Autodesk Inventor part; units mm, degrees
ref_plane "YZ Plane" through (0, 0, 0) normal (1, 0, 0) x (0, 1, 0)
ref_plane "XZ Plane" through (0, 0, 0) normal (0, 1, 0) x (-1, 0, 0)
ref_plane "XY Plane" through (0, 0, 0) normal (0, 0, 1) x (1, 0, 0)
sketch "Skizze1" plane through (0, 0, 0) normal (0, 1, 0) x (-1, 0, 0)
  line L0 (0, 0) -> (15, 0)
  line L1 (15, 0) -> (15, -17.5)
  line L2 (15, -17.5) -> (40, -17.5)
  line L3 (40, -17.5) -> (40, -47.5)
  line L4 (40, -47.5) -> (15, -47.5)
  line L5 (15, -47.5) -> (15, -65)
  line L6 (15, -65) -> (0, -65)
  line L7 (0, -65) -> (0, 0)
  dimension "d0" = 65
  dimension "d1" = 30
  dimension "d2" = 15
  dimension "d3" = 40
  dimension "d6" = 25
extrude "Extrusion3" add sketch "Skizze1" along normal blind 12
sketch "Skizze5" plane through (0, 0, 0) normal (0, -1, 0) x (1, 0, 0)
  line L0 (-7.5, -58) -> (-7.5, -43) construction
  line L1 (-4.95, -58) -> (-4.95, -43)
  line L2 (-10.05, -43) -> (-10.05, -58)
  arc A0 (-10.05, -58) -> (-4.95, -58) centre (-7.5, -58) ccw
  arc A1 (-4.95, -43) -> (-10.05, -43) centre (-7.5, -43) ccw
  line L3 (-7.5, -22) -> (-7.5, -7) construction
  line L4 (-4.95, -22) -> (-4.95, -7)
  line L5 (-10.05, -7) -> (-10.05, -22)
  arc A2 (-10.05, -22) -> (-4.95, -22) centre (-7.5, -22) ccw
  arc A3 (-4.95, -7) -> (-10.05, -7) centre (-7.5, -7) ccw
  line L6 (0, -65) -> (-15, -65)
  line L7 (-15, 0) -> (0, 0)
  line L8 (-15, -65) -> (-15, -47.5)
  line L9 (0, 0) -> (0, -65)
  point P0 (-7.5, -50.5)
  point P1 (-7.5, -14.5)
  dimension "d52" = 5.1
  dimension "d53" = 5.1
  dimension "d54" = 15
  dimension "d55" = 15
  dimension "d56" = 7
  dimension "d58" = 7
  dimension "d59" = 15
  dimension "d60" = 7.5
  dimension "d76" = 36
extrude "Extrusion5" cut sketch "Skizze5" against normal through all
sketch "Skizze6" plane through (0, 0, 0) normal (0, -1, 0) x (1, 0, 0)
  line L0 (-7.5, -58) -> (-7.5, -43) construction
  line L1 (-2.5, -58) -> (-2.5, -43)
  line L2 (-12.5, -43) -> (-12.5, -58)
  arc A0 (-12.5, -58) -> (-2.5, -58) centre (-7.5, -58) ccw
  arc A1 (-2.5, -43) -> (-12.5, -43) centre (-7.5, -43) ccw
  line L3 (-7.5, -22) -> (-7.5, -7) construction
  line L4 (-2.5, -22) -> (-2.5, -7)
  line L5 (-12.5, -7) -> (-12.5, -22)
  arc A2 (-12.5, -22) -> (-2.5, -22) centre (-7.5, -22) ccw
  arc A3 (-2.5, -7) -> (-12.5, -7) centre (-7.5, -7) ccw
  line L6 (-15, 0) -> (0, 0)
  line L7 (0, 0) -> (0, -65)
  point P0 (-7.5, -50.5)
  point P1 (-7.5, -14.5)
  dimension "d63" = 10
  dimension "d64" = 10
  dimension "d65" = 15
  dimension "d66" = 15
  dimension "d67" = 7
  dimension "d68" = 7.5
  dimension "d69" = 7.5
  dimension "d70" = 7
extrude "Extrusion6" cut sketch "Skizze6" against normal blind 5
fillet "Rundung4" radius 7.5 6 edges at (-15, 6, -65) (0, 6, -65) (0, 6, 0) (-15, 6, 0) (-15, 6, -17.5) (-15, 6, -47.5)
fillet "Rundung5" radius 15 2 edges at (-40, 6, -47.5) (-40, 6, -17.5)
sketch "Skizze7" plane through (0, 0, 0) normal (0, -1, 0) x (1, 0, 0)
  circle A0 centre (-30.5, -32.5) radius 3.7991
  point P0 (0, 0)
  dimension "d77" = 32.5
  dimension "d78" = 30.5
hole "Bohrung1" at (-30.5, 0, -32.5) direction (0, 1, 0) diameter 10.2 end through all counterbore diameter 17 counterbore depth 10
properties part number "Lampenhalterung1,0"
Design review of the part built by this model. Coordinates are the model's own, in mm. A direction names the side the tool comes from. Round coordinates to 2 decimals unless told otherwise and drop trailing zeros. Write each loop counter-clockwise with the first axis right and the second up, starting at its lowest first coordinate (ties: lowest second). Pieces come first, ordered by that corner, then holes.
Item 1: For pin 1 Ø11 at (x, z) = (-7.5, -8.5) entering from -Y; pin 2 Ø1.3 at (x, y) = (-24, 6.5) entering from +Z; pin 3 Ø6 at (x, y) = (-28.5, 3) entering from -Z; pin 4 Ø4 at (x, y) = (-31, 2) entering from +Z, all flat-tipped, find the tip position at first contact; note any pin that passes through.
Item 2: Draft analysis for pull direction X (two halves, no side actions). For faces 6 (the cylindrical face through (-17.255, 6.084, -49.639)), 7 (the cylindrical face through (-2.255, 6.084, -2.139)), 8 (the flat face through (-12.5, 2, -50)), state which applies: released by +X, released by -X, zero draft, split by the parting line, or undercut.
Item 3: Wall thickness on L1, parallel to X at y = 4.75, z = -39; L2, parallel to X at y = 11.5, z = -32.5; L3, parallel to X at y = 5, z = -32.5: over which ranges is each line inside the solid? List them lowest first.
Item 4: For faces 1 (the flat face through (-15, 12, -32)), 2 (the flat face through (-15, 6, -56)), 3 (the flat face through (-2.5, 2, -51)), 4 (the flat face through (-4.95, 8, -51)), 5 (the flat face through (-15, 6, -9)), list the 3-axis set-ups (+Z, -Z, +X, -X, +Y, -Y) from which the entire face can be reached by the end or side of a thin tool; tool diameter is ignored.
Item 5: Consider section B-B on x = -30.5. Give the boundary of the cut face in (y, z).
Item 6: Consider section C-C on z = -34. Give the boundary of the cut face in (x, y), and give its area (3 significant figures).
Item 7: Consider section A-A on y = 10.75. Count the separate pieces of the cut face and the enclosed holes in it, and give its area (3 significant figures).
Item 8: Consider section D-D on x = -4. Give the boundary of the cut face in (y, z).
Check values:
1. pin 1: stops at y = 0
1. pin 2: stops at z = -17.5
1. pin 3: stops at z = -47.49
1. pin 4: stops at z = -18.04
2. face 6: released by -X
2. face 7: released by +X
2. face 8: undercut
3. L1: x = -38.52 to -35.98, -25.02 to -10.5, -4.5 to 0
3. L2: x = -40 to -35.6, -25.4 to 0
3. L3: x = -40 to -39, -22 to 0
4. face 1: +Z, -Z, +X, -X, +Y
4. face 2: -Z, -X, +Y, -Y
4. face 3: -Y
4. face 4: +Y, -Y
4. face 5: +Z, -X, +Y, -Y
5. outline: (0, -46.46) - (12, -46.46) - (12, -37.6) - (10, -37.6) - (10, -41) - (0, -41) - close; (0, -24) - (10, -24) - (10, -27.4) - (12, -27.4) - (12, -18.54) - (0, -18.54) - close
6. outline: (-39.92, 0) - (-38.87, 0) - (-38.87, 10) - (-35.37, 10) - (-35.37, 12) - (-39.92, 12) - close; (-25.63, 10) - (-22.13, 10) - (-22.13, 0) - (0, 0) - (0, 12) - (-25.63, 12) - close
6. area: 292 mm2
7. separate pieces: 1
7. enclosed holes: 3
7. area: 1,330 mm2
8. outline: (0, -64.13) - (12, -64.13) - (12, -0.87) - (0, -0.87) - (0, -3.43) - (5, -3.43) - (5, -25.57) - (0, -25.57) - (0, -39.43) - (5, -39.43) - (5, -61.57) - (0, -61.57) - close
